Source: CAD feature listing. Evaluate the final solid. Frame: model axes, mm. Round coordinates to 2 decimals unless told otherwise and drop trailing zeros. Loops run counter-clockwise (first coordinate to the right, second up) from the corner with the lowest first, then second, coordinate; pieces in that order, holes last.
(1) Section B-B, the plane x = 0. Return the cut outline in (y, z), plus the area to 3 significant figures.
(2) First-contact query: pin 1 Ø10 at (x, z) = (-2, 2) entering from +Y; pin 2 Ø7 at (x, z) = (0, 0) entering from +Y. Flat tips, straight axial feed; report the tip coordinate or a pass-through.
(3) Mould query, pull axis X, two halves, no side actions, for faces 1 (the flat face through (3, 12, 4)), 2 (the cylindrical face through (-0.867, 5.916, -3.905)), 3 (the flat face through (16.5, 6, 0)). Classes: pulls with the +X half, pulls with the -X half, needs draft (parallel to the pull), parting line crosses it, or undercut.
(4) Material intervals for probe 1 along Z at (x, y) = (0, 6.5); probe 2 along Z at (x, y) = (1, 3.25), sorted ascending.
(5) Section A-A, the plane z = 0. Return the cut outline in (x, y).
(6) Section C-C, the plane y = 10.5. Return the cut outline in (x, z).
```python
from build123d import *

# Parameters (mm, degrees)
F0_W     = 33
F0_H     = 33
F1_DEPTH = 12
F2_R     = 4
F3_DEPTH = 12


with BuildPart() as f1:
    # F0 (on Front) → F1 (new body)
    with BuildSketch(Plane.XZ):
        Rectangle(F0_W, F0_H)
    extrude(amount=-F1_DEPTH)

    # F2 (on face) → F3 (cut)
    with BuildSketch(Plane.XZ):
        Circle(F2_R)
    extrude(amount=-F3_DEPTH, mode=Mode.SUBTRACT)


solid = f1.part
```
Output values:
1. outline: (0, -16.5) - (12, -16.5) - (12, -4) - (0, -4) - close; (0, 4) - (12, 4) - (12, 16.5) - (0, 16.5) - close
1. area: 300 mm2
2. pin 1: stops at y = 12
2. pin 2: passes through
3. face 1: needs draft
3. face 2: undercut
3. face 3: pulls with the +X half
4. probe 1: z = -16.5 to -4, 4 to 16.5
4. probe 2: z = -16.5 to -3.87, 3.87 to 16.5
5. outline: (-16.5, 0) - (-4, 0) - (-4, 12) - (-16.5, 12) - close; (4, 0) - (16.5, 0) - (16.5, 12) - (4, 12) - close
6. outline: (-16.5, -16.5) - (16.5, -16.5) - (16.5, 16.5) - (-16.5, 16.5) - close; hole circle Ø8 at (0, 0)
